Source: CAD feature listing. Evaluate the final solid. Frame: model axes, mm. A direction names the side the tool comes from. Coordinates: 2 decimals unless noted, no trailing zeros. Order: outer loops, then holes, each group sorted by start corner. A loop starts at its lowest first (then second) coordinate and runs counter-clockwise, first axis right, second up. Notation, with made-up numbers: (-24, 7.25) - (-10, 7.25) arc R28 ccw to (-10, 45.25) - close; hole circle Ø10 at (19.25, 5). An arc over 180 degrees is marked (long way). One line per question, with ' | ' between items. Start each with the question number.
(1) Section A-A (z = 50). Return the cut outline in (x, y).
(2) Section B-B (y = 436). Return the cut outline in (x, z), then the cut area to 3 significant figures.
(3) Access query for faces 4 (the flat face through (-1, 8, 0)), 5 (the cylindrical face through (-30, 8, 50)). Directions: +Z, -Z, +X, -X, +Y, -Y. A direction counts if a zero-diameter tool reaches every point of the face in a straight line with its end or side. Return the directions, or none.
(4) Draft query along Z for faces 1 (the flat face through (-1, -600, 27)), 2 (the flat face through (-1, 8, 100)), 3 (the flat face through (-40, 8, 50)). Return one class per face: +Z half, -Z half, draft (parallel to the pull), parting line (faces both ways), or undercut.
(5) Section C-C (x = 0). Return the cut outline in (y, z), then the cut area to 3 significant figures.
(6) Contact query for a flat-ended pin moving along its axis: P1, Ø24, axis at x = 0, z = 50, coming from the +Y side. Output: stop coordinate, or through.
(7) Line query: line 1 along X through (y, z) = (-164.5, 50); line 2 along X through (y, z) = (-414, 52.5); line 3 along Z through (x, y) = (27, -11). Output: solid intervals per line, ascending.
from build123d import *

# Parameters (mm, degrees)
SKETCH1_W           = 100
SKETCH1_H           = 1200
BOSS_EXTRUDE1_DEPTH = 100
SKETCH3_R           = 20
CUT_EXTRUDE1_DEPTH  = 1206.197079319


with BuildPart() as part:
    # Sketch1 → Boss-Extrude1 (new body)
    with BuildSketch(Plane.XY):
        Rectangle(SKETCH1_W, SKETCH1_H)
    extrude(amount=BOSS_EXTRUDE1_DEPTH)

    # Sketch3 → Cut-Extrude1 (cut, through all)
    with BuildSketch(Plane(origin=(0, 600, 0), x_dir=(1, 0, 0), z_dir=(0, 1, 0))):
        with Locations(Location((0, -50, 0), (0, 0, 270))):
            Circle(SKETCH3_R)
        with BuildLine():
            Line((-24.411222461, -67.438240105), (-40, -78.57413656))
            Line((-40, -78.57413656), (-40, -21.42586344))
            Line((-40, -21.42586344), (-24.411222461, -32.561759895))
            ThreePointArc((-24.411222461, -32.561759895), (-30, -50), (-24.411222461, -67.438240105))
        make_face()
        with BuildLine():
            Line((-17.438240105, -25.588777539), (-28.57413656, -10))
            Line((-28.57413656, -10), (28.57413656, -10))
            Line((28.57413656, -10), (17.438240105, -25.588777539))
            ThreePointArc((17.438240105, -25.588777539), (0, -20), (-17.438240105, -25.588777539))
        make_face()
        with BuildLine():
            Line((24.411222461, -32.561759895), (40, -21.42586344))
            Line((40, -21.42586344), (40, -78.57413656))
            Line((40, -78.57413656), (24.411222461, -67.438240105))
            ThreePointArc((24.411222461, -67.438240105), (30, -50), (24.411222461, -32.561759895))
        make_face()
        with BuildLine():
            Line((17.438240105, -74.411222461), (28.57413656, -90))
            Line((28.57413656, -90), (-28.57413656, -90))
            Line((-28.57413656, -90), (-17.438240105, -74.411222461))
            ThreePointArc((-17.438240105, -74.411222461), (0, -80), (17.438240105, -74.411222461))
        make_face()
    extrude(amount=-CUT_EXTRUDE1_DEPTH, mode=Mode.SUBTRACT)


solid = part.part
Response values:
1) outline: (-50, -600) - (-40, -600) - (-40, 600) - (-50, 600) - close; (-30, -600) - (-20, -600) - (-20, 600) - (-30, 600) - close; (20, -600) - (30, -600) - (30, 600) - (20, 600) - close; (40, -600) - (50, -600) - (50, 600) - (40, 600) - close
2) outline: (-50, 0) - (50, 0) - (50, 100) - (-50, 100) - close; hole (-40, 21.43) - (-24.41, 32.56) arc R30 cw to (-24.41, 67.44) - (-40, 78.57) - close; hole (-28.57, 10) - (28.57, 10) - (17.44, 25.59) arc R30 cw to (-17.44, 25.59) - close; hole (-28.57, 90) - (-17.44, 74.41) arc R30 cw to (17.44, 74.41) - (28.57, 90) - close; hole circle Ø40 at (0, 50); hole (24.41, 32.56) - (40, 21.43) - (40, 78.57) - (24.41, 67.44) arc R30 cw to start | area: 6,400 mm²
3) face 4: -Z, +X, -X, +Y, -Y | face 5: +Y, -Y
4) face 1: draft | face 2: +Z half | face 3: undercut
5) outline: (-600, 0) - (600, 0) - (600, 10) - (-600, 10) - close; (-600, 20) - (600, 20) - (600, 30) - (-600, 30) - close; (-600, 70) - (600, 70) - (600, 80) - (-600, 80) - close; (-600, 90) - (600, 90) - (600, 100) - (-600, 100) - close | area: 48,000 mm²
6) P1: passes through
7) line 1: x = -50 to -40, -30 to -20, 20 to 30, 40 to 50 | line 2: x = -50 to -40, -29.9 to -19.84, 19.84 to 29.9, 40 to 50 | line 3: z = 0 to 10, 12.2 to 30.71, 36.92 to 63.08, 69.29 to 87.8, 90 to 100
